Read the model definition and answer for the solid it produces. Units are mm, in the model's axes. Face numbers are marked on the shaded views. A direction names the side the tool comes from. Coordinates: 2 decimals unless noted, no trailing zeros. Order: outer loops, then holes, each group sorted by start corner. A loop starts at its lowest first (then second) coordinate and runs counter-clockwise, first axis right, second up. Notation, with made-up numbers: (17, 46) -> (42, 46) arc R21 ccw to (42, 64) -> close; hole circle Ø11 at (64.5, 32.25). An arc over 180 degrees is marked (long way). Answer as a JSON object with one key per item and string values. Group by question number.
1) Section D-D on y = 17 is taken. Determine the outline of the cut face in (x, z), and give its area (3 significant figures).
2) A tool of negligible diameter and unlimited length cuts with its end or side. For the marked faces 1, 2, 3 and 4, from which of +Z, -Z, +X, -X, +Y, -Y can it reach the whole face along a straight path? Write none if from no direction.
3) Section A-A on x = 0 is taken. Determine the outline of the cut face in (y, z).
4) Consider L1, parallel to Z at x = -75.5, y = 49.5; L2, parallel to X at y = 25, z = -29; L3, parallel to X at y = 1.7, z = -64.5. Determine where each line is inside the solid, lowest interval first.
5) Section C-C on y = 44 is taken. Determine the outline of the cut face in (x, z).
6) Determine the mould class of the marked faces 5, 6 and 7 for opening direction X: released by +X, released by -X, zero draft, split by the parting line, or undercut.
7) Given pin 1 (8 mm diameter, centred on x = -68.23, z = 65.5, fed in from +Y); pin 2 (12 mm diameter, centred on y = 50.5, z = 36.5, fed in from -X); pin 3 (6 mm diameter, centred on x = -22.5, y = 45.5, fed in from -Z); pin 4 (13 mm diameter, centred on x = -31, z = -63, fed in from +Y), each flat-ended and moving along its own axis, determine where each tip first touches the part or whether it passes through.
8) Section B-B on z = 65.5 is taken. Determine the outline of the cut face in (x, y).
from build123d import *

# Parameters (mm, degrees)
SKETCH_1_R          = 3
EXTRUDE_3_DEPTH     = 4
EXTRUDE_5_DEPTH     = 52
SKETCH_4_W          = 170
SKETCH_4_H          = 105
CUT_EXTRUDE_1_DEPTH = 52
FILLET_1_R          = 6
CUT_EXTRUDE_2_REACH = 205.755


with BuildPart() as part:
    # 草图1 → 凸台-拉伸3 (new body)
    with BuildSketch(Plane(origin=(0, 0, 0), x_dir=(1, 0, 0), z_dir=(0, 1, 0))):
        Polygon((-75, 70.5), (75, 70.5), (91, 52.5), (91, -52.5), (75, -72.5), (-75, -72.5), (-91, -52.5), (-91, 52.5), align=None)
        with Locations(Location((0, 64.5, 0), (0, 0, 270))):
            Circle(SKETCH_1_R, mode=Mode.SUBTRACT)
        with Locations(Location((-68.230807573, 64.5, 0), (0, 0, 270))):
            Circle(SKETCH_1_R, mode=Mode.SUBTRACT)
        with Locations(Location((70.140932989, 64.5, 0), (0, 0, 270))):
            Circle(SKETCH_1_R, mode=Mode.SUBTRACT)
        with Locations(Location((0, -65.5, 0), (0, 0, 270))):
            Circle(SKETCH_1_R, mode=Mode.SUBTRACT)
        with Locations(Location((70.140932989, -65.5, 0), (0, 0, 270))):
            Circle(SKETCH_1_R, mode=Mode.SUBTRACT)
        with Locations(Location((-68.230807573, -65.5, 0), (0, 0, 270))):
            Circle(SKETCH_1_R, mode=Mode.SUBTRACT)
    extrude(amount=EXTRUDE_3_DEPTH)

    # 草图3 → 凸台-拉伸5 (add)
    with BuildSketch(Plane(origin=(0, 4, 0), x_dir=(1, 0, 0), z_dir=(0, 1, 0))):
        Polygon((-91, 52.5), (-91, -52.5), (-86.2, -58.5), (86.2, -58.5), (91, -52.5), (91, 52.5), (85.666666667, 58.5), (-85.666666667, 58.5), align=None)
    extrude(amount=EXTRUDE_5_DEPTH)

    # 草图4 → 切除-拉伸1 (cut)
    with BuildSketch(Plane.XZ):
        Rectangle(SKETCH_4_W, SKETCH_4_H)
    extrude(amount=-CUT_EXTRUDE_1_DEPTH, mode=Mode.SUBTRACT)

    # 圆角1
    # the kernel refuses this fillet: 6 mm, written as the material it takes off along each edge
    with BuildSketch(Plane(origin=(-100.370425713, 56, 40.786967858), x_dir=(0.7808688094430221, 0, -0.6246950475544346), z_dir=(0.6246950475544346, 0, 0.7808688094430221)), Plane(origin=(76.829574287, 56, 70.213032142), x_dir=(-0.7808688094430356, 0, -0.6246950475544176), z_dir=(0.6246950475544177, 0, -0.7808688094430356))) as fillet_1_piece_1:
        with BuildLine():
            CenterArc((FILLET_1_R, -FILLET_1_R), FILLET_1_R, 90, 90)
            Line((0, -FILLET_1_R), (0, 0))
            Line((0, 0), (FILLET_1_R, 0))
        make_face()
    extrude(amount=37.683749085, mode=Mode.SUBTRACT)
    with BuildSketch(Plane(origin=(-75.701209084, 56, -69.71113978), x_dir=(0, -1, 0), z_dir=(-0.6643638388299179, 0, 0.7474093186836614))) as fillet_1_piece_2:
        with BuildLine():
            CenterArc((FILLET_1_R, FILLET_1_R), FILLET_1_R, 180, 90)
            Line((0, FILLET_1_R), (0, 0))
            Line((0, 0), (FILLET_1_R, 0))
        make_face()
    extrude(amount=38.027729719, mode=Mode.SUBTRACT)
    with BuildSketch(Plane(origin=(100.666666667, 56, -58.5), x_dir=(0, 0, 1), z_dir=(-1, 0, 0))) as fillet_1_piece_3:
        with BuildLine():
            CenterArc((FILLET_1_R, -FILLET_1_R), FILLET_1_R, 90, 90)
            Line((0, -FILLET_1_R), (0, 0))
            Line((0, 0), (FILLET_1_R, 0))
        make_face()
    extrude(amount=201.333333333, mode=Mode.SUBTRACT)
    with BuildSketch(Plane(origin=(91, 56, 67.5), x_dir=(-1, 0, 0), z_dir=(0, 0, -1))) as fillet_1_piece_4:
        with BuildLine():
            CenterArc((FILLET_1_R, -FILLET_1_R), FILLET_1_R, 90, 90)
            Line((0, -FILLET_1_R), (0, 0))
            Line((0, 0), (FILLET_1_R, 0))
        make_face()
    extrude(amount=135, mode=Mode.SUBTRACT)
    with BuildSketch(Plane(origin=(-91, 56, -67.5), x_dir=(0, -1, 0), z_dir=(0, 0, 1))) as fillet_1_piece_5:
        with BuildLine():
            CenterArc((FILLET_1_R, FILLET_1_R), FILLET_1_R, 180, 90)
            Line((0, FILLET_1_R), (0, 0))
            Line((0, 0), (FILLET_1_R, 0))
        make_face()
    extrude(amount=135, mode=Mode.SUBTRACT)
    with BuildSketch(Plane(origin=(-101.2, 56, 58.5), x_dir=(0, 0, -1), z_dir=(1, 0, 0))) as fillet_1_piece_6:
        with BuildLine():
            CenterArc((FILLET_1_R, -FILLET_1_R), FILLET_1_R, 90, 90)
            Line((0, -FILLET_1_R), (0, 0))
            Line((0, 0), (FILLET_1_R, 0))
        make_face()
    extrude(amount=202.4, mode=Mode.SUBTRACT)

    # 草图5 → 切除-拉伸2 (cut, up to next)
    with BuildSketch(Plane.ZY.offset(91), mode=Mode.PRIVATE) as cut_extrude_2_sk1:
        with BuildLine():
            Line((-25, 0), (25, 0))
            Line((25, 0), (25, 35))
            ThreePointArc((25, 35), (23.535533906, 38.535533906), (20, 40))
            Line((20, 40), (-20, 40))
            ThreePointArc((-20, 40), (-23.535533906, 38.535533906), (-25, 35))
            Line((-25, 35), (-25, 0))
        make_face()
    cut_extrude_2_tool1 = extrude(cut_extrude_2_sk1.sketch, amount=-CUT_EXTRUDE_2_REACH, mode=Mode.PRIVATE) & part.part
    add(cut_extrude_2_tool1.solids().sort_by_distance((-91, 19.898145, 0))[0], mode=Mode.SUBTRACT)


solid = part.part
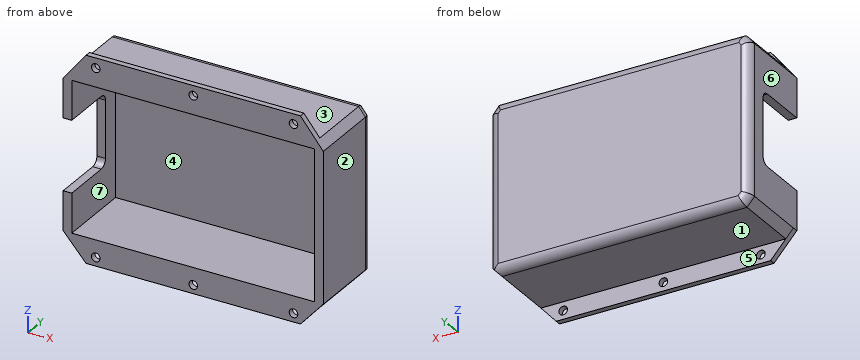
Worked answers:
{
 "1": {"outline": "(-91, -52.5) -> (-85.67, -58.5) -> (85.67, -58.5) -> (91, -52.5) -> (91, 52.5) -> (86.2, 58.5) -> (-86.2, 58.5) -> (-91, 52.5) -> (-91, 25) -> (-85, 25) -> (-85, 52.5) -> (85, 52.5) -> (85, -52.5) -> (-85, -52.5) -> (-85, -25) -> (-91, -25) -> close", "area": "3,080 mm²"},
 "2": {"face 1": "-Z, +X, -X, +Y", "face 2": "+Z, -Z, +X, +Y, -Y", "face 3": "+Z, +X, -X, +Y", "face 4": "-Y"},
 "3": {"outline": "(0, -70.5) -> (4, -70.5) -> (4, -67.5) -> (0, -67.5) -> close; (0, -61.5) -> (4, -61.5) -> (4, -58.5) -> (50, -58.5) arc R6 ccw to (56, -52.5) -> (56, 52.5) arc R6 ccw to (50, 58.5) -> (4, 58.5) -> (4, 62.5) -> (0, 62.5) -> (0, 52.5) -> (52, 52.5) -> (52, -52.5) -> (0, -52.5) -> close; (0, 68.5) -> (4, 68.5) -> (4, 72.5) -> (0, 72.5) -> close"},
 "4": {"L1": "z = -58.5 to -52.5, 52.5 to 58.5", "L2": "x = -91 to -85, 85 to 91", "L3": "x = -80.33 to -71.23, -65.23 to -3, 3 to 67.14, 73.14 to 80.33"},
 "5": {"outline": "(-91, -52.5) -> (-85.67, -58.5) -> (85.67, -58.5) -> (91, -52.5) -> (91, 52.5) -> (86.2, 58.5) -> (-86.2, 58.5) -> (-91, 52.5) -> close; hole (-85, -52.5) -> (85, -52.5) -> (85, 52.5) -> (-85, 52.5) -> close"},
 "6": {"face 5": "zero draft", "face 6": "released by -X", "face 7": "undercut"},
 "7": {"pin 1": "stops at y = 4", "pin 2": "stops at x = -91", "pin 3": "stops at z = -58.5", "pin 4": "stops at y = 54.47"},
 "8": {"outline": "(-80.6, 0) -> (-71.23, 0) -> (-71.23, 4) -> (-80.6, 4) -> close; (-65.23, 0) -> (-3, 0) -> (-3, 4) -> (-65.23, 4) -> close; (3, 0) -> (67.14, 0) -> (67.14, 4) -> (3, 4) -> close; (73.14, 0) -> (80.6, 0) -> (80.6, 4) -> (73.14, 4) -> close"}
}
